```python
from build123d import *

# Parameters (mm, degrees)
SKETCH_2_W          = 80
SKETCH_2_H          = 50
SKETCH_2_R          = 2.65
EXTRUDE_1_DEPTH     = 2
SKETCH_3_W          = 2.5
SKETCH_3_H          = 35
SKETCH_3_W_2        = 17
SKETCH_3_H_2        = 2.5
EXTRUDE_2_DEPTH     = 30
CUT_EXTRUDE_1_REACH = 61.691
SKETCH_4_R          = 1.35
SKETCH_4_W          = 5.2
SKETCH_4_H          = 17
FILLET_1_R          = 2
FILLET_2_R          = 1
CUT_EXTRUDE_2_DEPTH = 67.560123197


with BuildPart() as part:
    # 草图2 → 凸台-拉伸1 (new body)
    with BuildSketch(Plane(origin=(0, 0, 0), x_dir=(1, 0, 0), z_dir=(0, 1, 0))):
        Rectangle(SKETCH_2_W, SKETCH_2_H)
        with Locations(Location((-30, 20, 0), (0, 0, 270))):
            Circle(SKETCH_2_R, mode=Mode.SUBTRACT)
        with Locations(Location((30, 20, 0), (0, 0, 90))):
            Circle(SKETCH_2_R, mode=Mode.SUBTRACT)
        with Locations(Location((-30, -20, 0), (0, 0, 90))):
            Circle(SKETCH_2_R, mode=Mode.SUBTRACT)
        with Locations(Location((30, -20, 0), (0, 0, 270))):
            Circle(SKETCH_2_R, mode=Mode.SUBTRACT)
    extrude(amount=EXTRUDE_1_DEPTH)

    # 草图3 → 凸台-拉伸2 (add)
    with BuildSketch(Plane(origin=(0, 2, 0), x_dir=(1, 0, 0), z_dir=(0, 1, 0))):
        with Locations((5, 0)):
            Rectangle(SKETCH_3_W, SKETCH_3_H)
        with Locations((14.75, 16.25)):
            Rectangle(SKETCH_3_W_2, SKETCH_3_H_2)
        with Locations((14.75, -16.25)):
            Rectangle(SKETCH_3_W_2, SKETCH_3_H_2)
    extrude(amount=EXTRUDE_2_DEPTH)

    # 草图4 → 切除-拉伸1 (cut, up to next)
    with BuildSketch(Plane.ZY.offset(-3.75), mode=Mode.PRIVATE) as cut_extrude_1_sk1:
        with Locations((11, 17)):
            Circle(SKETCH_4_R)
    cut_extrude_1_tool1 = extrude(cut_extrude_1_sk1.sketch, amount=-CUT_EXTRUDE_1_REACH, mode=Mode.PRIVATE) & part.part
    # 草图4 → 切除-拉伸1 (cut, up to next)
    with BuildSketch(Plane.ZY.offset(-3.75), mode=Mode.PRIVATE) as cut_extrude_1_sk2:
        with Locations((-11, 17)):
            Circle(SKETCH_4_R)
    cut_extrude_1_tool2 = extrude(cut_extrude_1_sk2.sketch, amount=-CUT_EXTRUDE_1_REACH, mode=Mode.PRIVATE) & part.part
    # 草图4 → 切除-拉伸1 (cut, up to next)
    with BuildSketch(Plane.ZY.offset(-3.75), mode=Mode.PRIVATE) as cut_extrude_1_sk3:
        with Locations((0, 23.5)):
            Rectangle(SKETCH_4_W, SKETCH_4_H)
    cut_extrude_1_tool3 = extrude(cut_extrude_1_sk3.sketch, amount=-CUT_EXTRUDE_1_REACH, mode=Mode.PRIVATE) & part.part
    # 草图4 → 切除-拉伸1 (cut, up to next)
    with BuildSketch(Plane.ZY.offset(-3.75), mode=Mode.PRIVATE) as cut_extrude_1_sk4:
        with BuildLine():
            Line((-2.6, 15), (2.6, 15))
            ThreePointArc((2.6, 15), (0, 12.4), (-2.6, 15))
        make_face()
    cut_extrude_1_tool4 = extrude(cut_extrude_1_sk4.sketch, amount=-CUT_EXTRUDE_1_REACH, mode=Mode.PRIVATE) & part.part
    add(cut_extrude_1_tool1.solids().sort_by_distance((3.75, 17, 11))[0], mode=Mode.SUBTRACT)
    add(cut_extrude_1_tool2.solids().sort_by_distance((3.75, 17, -11))[0], mode=Mode.SUBTRACT)
    add(cut_extrude_1_tool3.solids().sort_by_distance((3.75, 23.5, 0))[0], mode=Mode.SUBTRACT)
    add(cut_extrude_1_tool4.solids().sort_by_distance((3.75, 13.896526, 0))[0], mode=Mode.SUBTRACT)

    # 圆角1
    # the kernel refuses this fillet: 2 mm, written as the material it takes off along each edge
    with BuildSketch(Plane(origin=(6.25, 37, 2.6), x_dir=(0, 0, 1), z_dir=(0, -1, 0)), Plane(origin=(6.25, 15, -2.6), x_dir=(0, 0, -1), z_dir=(0, 1, 0)), Plane(origin=(3.75, 37, -2.6), x_dir=(0, 0, -1), z_dir=(0, -1, 0)), Plane(origin=(3.75, 15, 2.6), x_dir=(0, 0, 1), z_dir=(0, 1, 0))) as fillet_1_piece_1:
        with BuildLine():
            CenterArc((FILLET_1_R, FILLET_1_R), FILLET_1_R, 180, 90)
            Line((0, FILLET_1_R), (0, 0))
            Line((0, 0), (FILLET_1_R, 0))
        make_face()
    extrude(amount=22, mode=Mode.SUBTRACT)
    with BuildSketch(Plane(origin=(6.25, 15, 0), x_dir=(0, 0, -1), z_dir=(0, 1, 0))) as fillet_1_piece_2:
        with BuildLine():
            CenterArc((2.6 + FILLET_1_R, FILLET_1_R), FILLET_1_R, 180, 90)
            Line((2.6, FILLET_1_R), (2.6, 0))
            Line((2.6, 0), (2.6 + FILLET_1_R, 0))
        make_face()
    revolve(axis=Axis((6.25, 15, 0), (-1, 0, 0)), revolution_arc=180, mode=Mode.SUBTRACT)
    with BuildSketch(Plane(origin=(3.75, 15, 0), x_dir=(0, 0, 1), z_dir=(0, 1, 0))) as fillet_1_piece_3:
        with BuildLine():
            CenterArc((2.6 + FILLET_1_R, FILLET_1_R), FILLET_1_R, 180, 90)
            Line((2.6, FILLET_1_R), (2.6, 0))
            Line((2.6, 0), (2.6 + FILLET_1_R, 0))
        make_face()
    revolve(axis=Axis((3.75, 15, 0), (1, 0, 0)), revolution_arc=180, mode=Mode.SUBTRACT)
    with BuildSketch(Plane(origin=(3.75, 2, -17.5), x_dir=(1, 0, 0), z_dir=(0, 1, 0))) as fillet_1_piece_4:
        with BuildLine():
            CenterArc((FILLET_1_R, -FILLET_1_R), FILLET_1_R, 90, 90)
            Line((0, -FILLET_1_R), (0, 0))
            Line((0, 0), (FILLET_1_R, 0))
        make_face()
    extrude(amount=35, mode=Mode.SUBTRACT)
    with BuildSketch(Plane(origin=(3.75, 2, 17.5), x_dir=(1, 0, 0), z_dir=(0, 1, 0))) as fillet_1_piece_5:
        with BuildLine():
            CenterArc((FILLET_1_R, FILLET_1_R), FILLET_1_R, 180, 90)
            Line((0, FILLET_1_R), (0, 0))
            Line((0, 0), (FILLET_1_R, 0))
        make_face()
    extrude(amount=35, mode=Mode.SUBTRACT)
    # the kernel refuses this fillet: 2 mm, written as the material it adds along each edge
    with BuildSketch(Plane(origin=(5.75, 2, 17.5), x_dir=(0, 0, 1), z_dir=(1, 0, 0))) as fillet_1_2_piece_1:
        with BuildLine():
            CenterArc((FILLET_1_R, -FILLET_1_R), FILLET_1_R, 90, 90)
            Line((0, -FILLET_1_R), (0, 0))
            Line((0, 0), (FILLET_1_R, 0))
        make_face()
    extrude(amount=17.5)
    with BuildSketch(Plane(origin=(5.75, 2, -17.5), x_dir=(0, 0, -1), z_dir=(1, 0, 0))) as fillet_1_2_piece_2:
        with BuildLine():
            CenterArc((FILLET_1_R, FILLET_1_R), FILLET_1_R, 180, 90)
            Line((0, FILLET_1_R), (0, 0))
            Line((0, 0), (FILLET_1_R, 0))
        make_face()
    extrude(amount=17.5)
    with BuildSketch(Plane(origin=(3.75, 2, -15.5), x_dir=(-1, 0, 0), z_dir=(0, 0, 1))) as fillet_1_2_piece_3:
        with BuildLine():
            CenterArc((FILLET_1_R, -FILLET_1_R), FILLET_1_R, 90, 90)
            Line((0, -FILLET_1_R), (0, 0))
            Line((0, 0), (FILLET_1_R, 0))
        make_face()
    extrude(amount=31)
    with BuildSketch(Plane(origin=(5.75, 2, -15.5), x_dir=(0, 0, -1), z_dir=(1, 0, 0))) as fillet_1_2_piece_4:
        with BuildLine():
            CenterArc((2 + FILLET_1_R, FILLET_1_R), FILLET_1_R, 180, 90)
            Line((2, FILLET_1_R), (2, 0))
            Line((2, 0), (2 + FILLET_1_R, 0))
        make_face()
    revolve(axis=Axis((5.75, 2, -15.5), (0, 1, 0)), revolution_arc=90)
    with BuildSketch(Plane(origin=(5.75, 2, 15.5), x_dir=(0, 0, 1), z_dir=(1, 0, 0))) as fillet_1_2_piece_5:
        with BuildLine():
            CenterArc((2 + FILLET_1_R, -FILLET_1_R), FILLET_1_R, 90, 90)
            Line((2, -FILLET_1_R), (2, 0))
            Line((2, 0), (2 + FILLET_1_R, 0))
        make_face()
    revolve(axis=Axis((5.75, 2, 15.5), (0, -1, 0)), revolution_arc=90)

    # 圆角2
    fillet_2_edges = [part.edges().sort_by_distance(p)[0] for p in [
        (-40, 2, 0),
        (0, 2, 25),
        (40, 2, 0),
        (0, 2, -25),
    ]]
    fillet(fillet_2_edges, radius=FILLET_2_R)

    # 草图5 → 切除-拉伸2 (cut, through all)
    with BuildSketch(Plane.XY.offset(17.5)):
        with BuildLine():
            Line((23.25, 32), (6.25, 32))
            add(Edge.make_bspline(
                [(6.25, 32), (16.534964458, 27.088669385), (23.25, 17.881434401), (23.25, 4)],
                knots=[0, 0, 0, 0, 1, 1, 1, 1], degree=3))
            Line((23.25, 4), (23.25, 32))
        make_face()
    extrude(amount=-CUT_EXTRUDE_2_DEPTH, mode=Mode.SUBTRACT)


solid = part.part
```
Work out the finished part from the listing and answer in its coordinate system (mm). A direction names the side the tool comes from. Give positions to 0.01 mm unless a question says otherwise; leave off trailing zeros. Order: outer loops, then holes, each group sorted by start corner. A loop starts at its lowest first (then second) coordinate and runs counter-clockwise, first axis right, second up. Notation, with made-up numbers: (4.5, 72) - (10.5, 72) arc R23 cw to (10.5, 97) - close; hole circle Ø3 at (-5.5, 4.25). An arc over 180 degrees is marked (long way). One line per item, written item: value. Start each with the question number.
1. Each of these flat-tipped pins is pushed along its axis until it touches: pin 1 Ø3 at (y, z) = (4.5, 17) entering from +X; pin 2 Ø3.5 at (y, z) = (17, 11) entering from +X; pin 3 Ø1.5 at (y, z) = (16, -14.5) entering from -X. Where does it stop, or does it pass through?
2. Section D-D, the plane z = 10.5 is taken. Write down the section's boundary in (x, y), then the cut area to 3 significant figures.
3. Section C-C, the plane z = 21.5 is taken. Write down the section's boundary in (x, y), then the cut area to 3 significant figures.
4. Section A-A, the plane x = -30 is taken. Write down the section's boundary in (y, z).
5. Consider line 1 (Y direction, x = 5, z = 11); line 2 (X direction, y = 1.2, z = 20); line 3 (Z direction, x = 16.5, y = 14). Determine where each line is inside the solid, lowest interval first.
6. For a pull along Z with two mould halves and no side action, classify faces 1 (the face through (-27.766, 0.986, -18.575)), 2 (the face through (12, 15, 17.5)), 3 (the face through (13, 15, -17.5)), 4 (the face through (4.1, 23.62, -3.47)) as released by +Z, released by -Z, zero draft, split by the parting line, or undercut.
7. Section B-B, the plane z = -11 is taken. Write down the section's boundary in (x, y).
8. Which of the six approach directions +Z, -Z, +X, -X, +Y, -Y give full straight-line access (tool end or side, diameter ignored) to faces 5 (the face through (23.25, 3, 16)), 6 (the face through (4.32, 17.8, 16.9)), 7 (the face through (5.9, 23.38, -3.47))?
Filled sheet:
1. pin 1: x = 23.25
1. pin 2: x = 6.25
1. pin 3: x = 3.75
2. outline: (-40, 0) - (40, 0) - (40, 1) arc R1 ccw to (39, 2) - (6.25, 2) - (6.25, 15.75) - (3.75, 15.75) - (3.75, 4) arc R2 cw to (1.75, 2) - (-39, 2) arc R1 ccw to (-40, 1) - close; (3.75, 18.25) - (6.25, 18.25) - (6.25, 32) - (3.75, 32) - close
2. area: 229 mm²
3. outline: (-40, 0) - (-32.18, 0) - (-32.18, 2) - (-39, 2) arc R1 ccw to (-40, 1) - close; (-27.82, 0) - (27.82, 0) - (27.82, 2) - (-27.82, 2) - close; (32.18, 0) - (40, 0) - (40, 1) arc R1 ccw to (39, 2) - (32.18, 2) - close
3. area: 142 mm²
4. outline: (0, -25) - (1, -25) arc R1 ccw to (2, -24) - (2, -22.65) - (0, -22.65) - close; (0, -17.35) - (2, -17.35) - (2, 17.35) - (0, 17.35) - close; (0, 22.65) - (2, 22.65) - (2, 24) arc R1 ccw to (1, 25) - (0, 25) - close
5. line 1: 0 to 15.65, 18.35 to 32
5. line 2: -39.98 to -32.65, -27.35 to 27.35, 32.65 to 39.98
5. line 3: -17.5 to -15, 15 to 17.5
6. face 1: undercut
6. face 2: released by +Z
6. face 3: released by -Z
6. face 4: undercut
7. outline: (-40, 0) - (40, 0) - (40, 1) arc R1 ccw to (39, 2) - (6.25, 2) - (6.25, 15.65) - (3.75, 15.65) - (3.75, 4) arc R2 cw to (1.75, 2) - (-39, 2) arc R1 ccw to (-40, 1) - close; (3.75, 18.35) - (6.25, 18.35) - (6.25, 32) - (3.75, 32) - close
8. face 5: +Z, -Z, +X, +Y
8. face 6: +Z, -X, +Y
8. face 7: +X, +Y
